For this review, use the dimensioned drawing (mm, ordinates from the lowest corner) and the shaded views. Coordinates: 2 decimals unless noted, no trailing zeros. Loops run counter-clockwise (first coordinate to the right, second up) from the corner with the lowest first, then second, coordinate; pieces in that order, holes last. Notation, with made-up numbers: (0, 59) - (25, 59) arc R24 ccw to (25, 72) - close; hole circle Ø7 at (-22.75, 61.25). An arc over 180 degrees is marked (long way). Answer in a Markdown table with one row per item. Add a question column.
(1) We need section C-C, the plane z = 158. Write out the cut boundary in (x, y).
(2) We need section B-B, the plane x = 59. Write out the cut boundary in (y, z), plus the area to 3 significant figures.
(3) We need section D-D, the plane x = 143. Write out the cut boundary in (y, z), plus the area to 3 significant figures.
(4) To check wall thickness, follow L1, parallel to Z at x = 9.5, y = 40.5; L2, parallel to X at y = 172, z = 161.5; L3, parallel to Z at x = 37, y = 105. State the ranges of each line that lie inside material, in increasing order. Write a range as [from, to].
(5) We need section A-A, the plane y = 55. Write out the cut boundary in (x, z).
(6) Clearance check with flat-ended pins moving along their axes: pin 1 (4 mm diameter, centred on x = 37.5, y = 87, fed in from +Z); pin 2 (8 mm diameter, centred on x = 78, z = 185.5, fed in from -Y); pin 3 (6 mm diameter, centred on x = 128, y = 44, fed in from +Z); pin 4 (11 mm diameter, centred on y = 109.5, z = 182.5, fed in from +X). State where each tip first meets the part, or that it passes through.
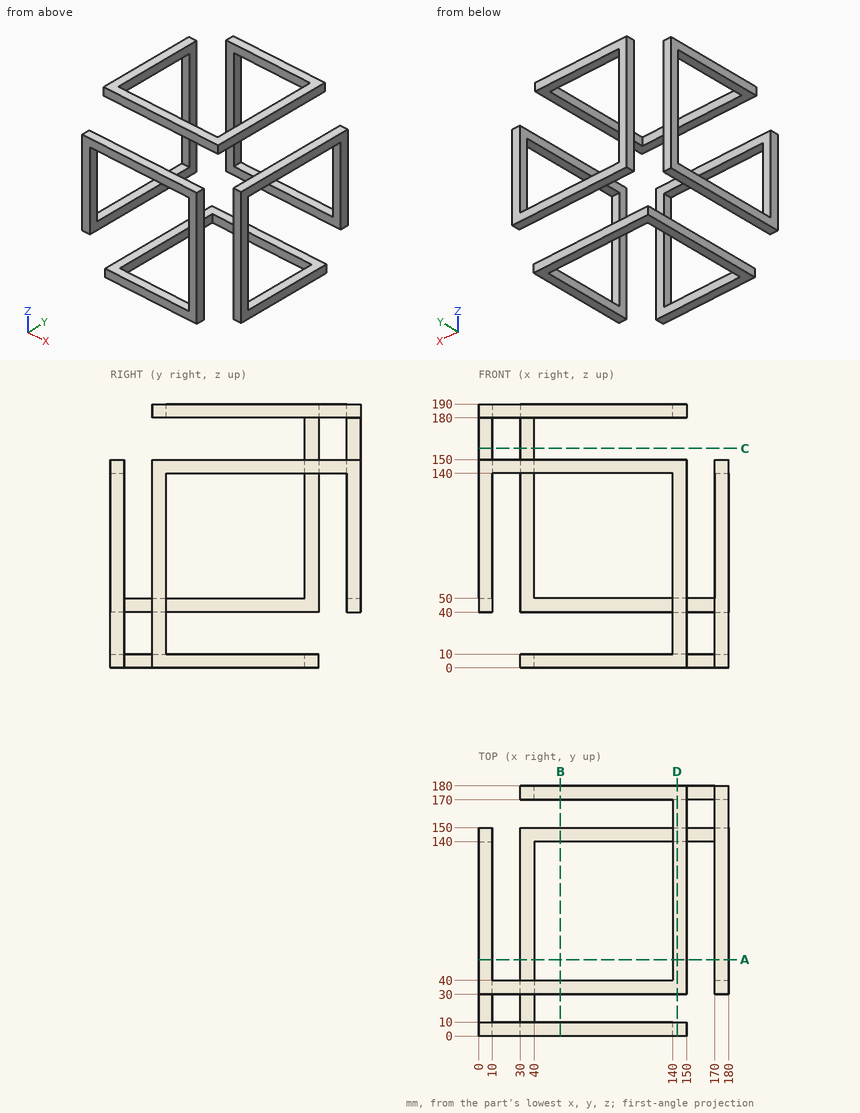
Responses:
| question | item | result |
|---|---|---|
| 1 | outline | (0, 140) - (10, 140) - (10, 150) - (0, 150) - close; (30, 170) - (40, 170) - (40, 180) - (30, 180) - close |
| 2 | outline | (0, 0) - (10, 0) - (10, 10) - (0, 10) - close; (0, 140) - (10, 140) - (10, 150) - (0, 150) - close; (30, 180) - (40, 180) - (40, 190) - (30, 190) - close; (140, 0) - (150, 0) - (150, 10) - (140, 10) - close; (170, 40) - (180, 40) - (180, 50) - (170, 50) - close; (170, 180) - (180, 180) - (180, 190) - (170, 190) - close |
| 2 | area | 600 mm2 |
| 3 | outline | (0, 0) - (10, 0) - (10, 150) - (0, 150) - close; (30, 180) - (180, 180) - (180, 190) - (30, 190) - close; (140, 0) - (150, 0) - (150, 10) - (140, 10) - close; (170, 40) - (180, 40) - (180, 50) - (170, 50) - close |
| 3 | area | 3,200 mm2 |
| 4 | L1 | z = [40, 50], [180, 190] |
| 4 | L2 | x = [30, 40] |
| 4 | L3 | z = [0, 10] |
| 5 | outline | (0, 40) - (10, 40) - (10, 50) - (0, 50) - close; (0, 180) - (10, 180) - (10, 190) - (0, 190) - close; (30, 0) - (40, 0) - (40, 10) - (30, 10) - close; (140, 180) - (150, 180) - (150, 190) - (140, 190) - close; (170, 0) - (180, 0) - (180, 10) - (170, 10) - close; (170, 140) - (180, 140) - (180, 150) - (170, 150) - close |
| 6 | pin 1 | stops at z = 10 |
| 6 | pin 2 | stops at y = 30 |
| 6 | pin 3 | passes through |
| 6 | pin 4 | stops at x = 150 |
